Geometry check sheet. Reference: the model listing, model coordinates, mm. Face numbers are marked on the shaded views. A direction names the side the tool comes from. Round coordinates to 2 decimals unless told otherwise and drop trailing zeros. Loops run counter-clockwise (first coordinate to the right, second up) from the corner with the lowest first, then second, coordinate; pieces in that order, holes last. Notation, with made-up numbers: M 59,87.5 L 76,87.5 A27 ccw 76,110.5 Z; hole C -29.5,81.25 d4. An arc over 180 degrees is marked long. Write item = value, one per line.
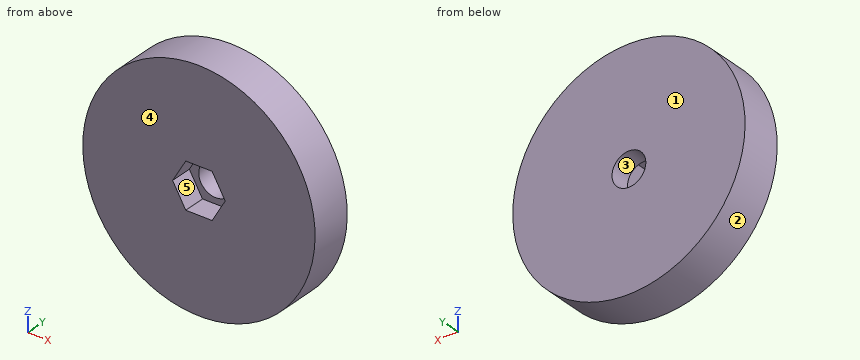
from build123d import *

# Parameters (mm, degrees)
SKETCH1_R              = 34.384
BOSS_EXTRUDE1_DEPTH    = 12.5
F_10_0MM_DOWEL_HOLE1_D = 10
CUT_EXTRUDE1_DEPTH     = 6.5


with BuildPart() as part:
    # Sketch1 → Boss-Extrude1 (new body)
    with BuildSketch(Plane(origin=(0, 0, 0), x_dir=(1, 0, 0), z_dir=(0, 1, 0))):
        with Locations(Location((0, 0, 0), (0, 0, 270))):
            Circle(SKETCH1_R)
    extrude(amount=BOSS_EXTRUDE1_DEPTH)

    # Ø10.0mm Dowel Hole1 (through all)
    with Locations(Plane(origin=(0, 0, 0), x_dir=(-1, 0, 0), z_dir=(0, -1, 0))):
        with Locations((0, 0)):
            Hole(F_10_0MM_DOWEL_HOLE1_D / 2)

    # Sketch4 → Cut-Extrude1 (cut)
    with BuildSketch(Plane(origin=(0, 0, 0), x_dir=(-1, 0, 0), z_dir=(0, -1, 0))):
        Polygon((-3.897114317, -6.75), (3.897114317, -6.75), (7.794228634, 0), (3.897114317, 6.75), (-3.897114317, 6.75), (-7.794228634, 0), align=None)
    extrude(amount=-CUT_EXTRUDE1_DEPTH, mode=Mode.SUBTRACT)


solid = part.part
(1) Material ranges on line 1 along Z through (x, y) = (-2.5, 12); line 2 along X through (y, z) = (4, -6); line 3 along X through (y, z) = (1.25, 6.5), recorded low to high. Write a range as from..to.
Result set:
line_1 = -34.29..-4.33, 4.33..34.29
line_2 = -33.86..-4.33, 4.33..33.86
line_3 = -33.76..-4.04, 4.04..33.76
(2) Sectioned sample at B-B on x = 0. Record the cut outline in (y, z), then the cut area to 3 significant figures.
Result set:
outline = M 0,-34.38 L 12.5,-34.38 L 12.5,-5 L 6.5,-5 L 6.5,-6.75 L 0,-6.75 Z; M 0,6.75 L 6.5,6.75 L 6.5,5 L 12.5,5 L 12.5,34.38 L 0,34.38 Z
area = 712 mm2
(3) Depth check by flat-ended pin: pin 1 Ø2 at (x, y) = (-2, 4.5) entering from +Z; pin 2 Ø5 at (y, z) = (10, -1) entering from -X; pin 3 Ø4 at (x, z) = (3.5, -2) entering from -Y; pin 4 Ø5 at (x, y) = (-1.5, 2) entering from -Z. Enter the tip coordinate at first touch or a pass-through.
Result set:
pin_1 = 34.37
pin_2 = -34.38
pin_3 = 6.5
pin_4 = -34.38
(4) Release check for a two-part mould opening along X. For the marked faces 1, 2 and 3 record: released by +X, released by -X, zero draft, split by the parting line, or undercut.
Result set:
face_1 = zero draft
face_2 = split by the parting line
face_3 = undercut
(5) Sectioned sample at A-A on z = -4. Record the cut outline in (x, y).
Result set:
outline = M -34.15,0 L -5.48,0 L -5.48,6.5 L -3,6.5 L -3,12.5 L -34.15,12.5 Z; M 3,6.5 L 5.48,6.5 L 5.48,0 L 34.15,0 L 34.15,12.5 L 3,12.5 Z
(6) Sectioned sample at C-C on y = 8.25. Record the cut outline in (x, z).
Result set:
outline = C 0,0 d68.77; hole C 0,0 d10
(7) Sectioned sample at D-D on x = -27.5. Record the cut outline in (y, z).
Result set:
outline = M 0,-20.64 L 12.5,-20.64 L 12.5,20.64 L 0,20.64 Z
(8) Tool access check on the marked faces 4 and 5. Record the directions out of +Z, -Z, +X, -X, +Y, -Y that give a thin tool (end or side, any length) a straight path to the whole face; none if there is none.
Result set:
face_4 = +Z, -Z, +X, -X, -Y
face_5 = -Y
